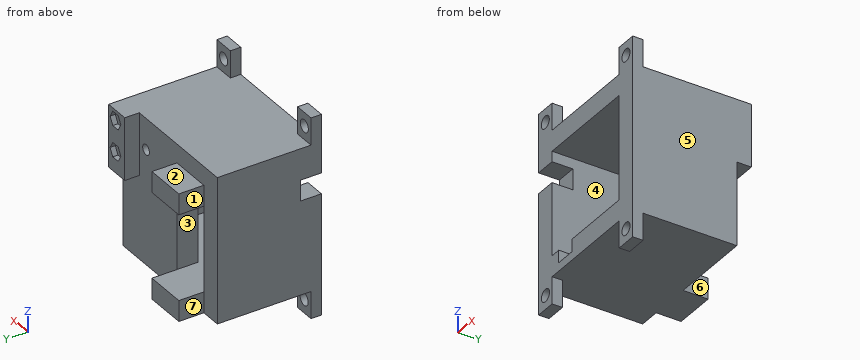
from build123d import *

# Parameters (mm, degrees)
SKETCH1_W               = 70
SKETCH1_H               = 70
BOSS_EXTRUDE1_DEPTH     = 50
CUT_EXTRUDE1_DEPTH      = 40
SKETCH3_W               = 20
SKETCH3_H               = 41
CUT_EXTRUDE2_DEPTH      = 40
SKETCH4_W               = 12
SKETCH4_H               = 30
BOSS_EXTRUDE2_DEPTH     = 7
CUT_EXTRUDE3_DEPTH      = 2.5
SKETCH7_R               = 2.5
CUT_EXTRUDE4_DEPTH      = 52.5
CUT_EXTRUDE5_DEPTH      = 97.81941954
CUT_EXTRUDE5_DEPTH_BACK = 52.5
SKETCH9_W               = 10
SKETCH9_H               = 10
SKETCH10_W              = 10
SKETCH10_H              = 6
CUT_EXTRUDE6_DEPTH      = 35
SKETCH11_W              = 20
SKETCH11_H              = 10
BOSS_EXTRUDE3_DEPTH     = 12
SKETCH13_W              = 10
SKETCH13_H              = 5
BOSS_EXTRUDE4_DEPTH     = 13
SKETCH14_W              = 10
SKETCH14_H              = 5
BOSS_EXTRUDE5_DEPTH     = 13
SKETCH15_R              = 3
CUT_EXTRUDE7_DEPTH      = 33


with BuildPart() as part:
    # Sketch1 → Boss-Extrude1 (new body)
    with BuildSketch(Plane(origin=(0, 0, 0), x_dir=(1, 0, 0), z_dir=(0, 1, 0))):
        Rectangle(SKETCH1_W, SKETCH1_H)
    extrude(amount=BOSS_EXTRUDE1_DEPTH)

    # Sketch2 → Cut-Extrude1 (cut)
    with BuildSketch(Plane.XZ):
        Polygon((0, 25), (-25, 25), (-25, -25), (25, -25), (25, 25), align=None)
    extrude(amount=-CUT_EXTRUDE1_DEPTH, mode=Mode.SUBTRACT)

    # Sketch3 → Cut-Extrude2 (cut)
    with BuildSketch(Plane(origin=(0, 50, 0), x_dir=(1, 0, 0), z_dir=(0, 1, 0))):
        with Locations((-15, 4.5)):
            Rectangle(SKETCH3_W, SKETCH3_H)
    extrude(amount=-CUT_EXTRUDE2_DEPTH, mode=Mode.SUBTRACT)

    # Sketch4 → Boss-Extrude2 (add)
    with BuildSketch(Plane(origin=(0, 50, 0), x_dir=(1, 0, 0), z_dir=(0, 1, 0))):
        with Locations((29, -20)):
            Rectangle(SKETCH4_W, SKETCH4_H)
    extrude(amount=BOSS_EXTRUDE2_DEPTH)

    # Sketch5 → Cut-Extrude3 (cut)
    with BuildSketch(Plane(origin=(0, 57, 0), x_dir=(1, 0, 0), z_dir=(0, 1, 0))):
        Polygon((33.881686691, -15), (31.881686691, -18.464101615), (27.881686691, -18.464101615), (25.881686691, -15), (27.881686691, -11.535898385), (31.881686691, -11.535898385), align=None)
        Polygon((27.881686691, -33.464101615), (25.881686691, -30), (27.881686691, -26.535898385), (31.881686691, -26.535898385), (33.881686691, -30), (31.881686691, -33.464101615), align=None)
    extrude(amount=-CUT_EXTRUDE3_DEPTH, mode=Mode.SUBTRACT)

    # Sketch7 → Cut-Extrude4 (cut)
    with BuildSketch(Plane(origin=(0, 50, 0), x_dir=(1, 0, 0), z_dir=(0, 1, 0))):
        with Locations(Location((18, -20, 0), (0, 0, 270))):
            Circle(SKETCH7_R)
    extrude(amount=-CUT_EXTRUDE4_DEPTH, mode=Mode.SUBTRACT)

    # Sketch9 → Cut-Extrude5 (cut, two sides: drawn at the far end of the back side and taken through both)
    with BuildSketch(Plane.ZY.offset(35).offset(-CUT_EXTRUDE5_DEPTH_BACK)):
        with Locations((15, 5)):
            Rectangle(SKETCH9_W, SKETCH9_H)
    extrude(amount=CUT_EXTRUDE5_DEPTH + CUT_EXTRUDE5_DEPTH_BACK, mode=Mode.SUBTRACT)

    # Sketch10 → Cut-Extrude6 (cut)
    with BuildSketch(Plane.XZ):
        with Locations((-15, -28)):
            Rectangle(SKETCH10_W, SKETCH10_H)
    extrude(amount=-CUT_EXTRUDE6_DEPTH, mode=Mode.SUBTRACT)

    # Sketch11 → Boss-Extrude3 (add)
    with BuildSketch(Plane(origin=(0, 50, 0), x_dir=(1, 0, 0), z_dir=(0, 1, 0))):
        with Locations((-15, 30)):
            Rectangle(SKETCH11_W, SKETCH11_H)
        with Locations((-15, -21)):
            Rectangle(SKETCH11_W, SKETCH11_H)
    extrude(amount=BOSS_EXTRUDE3_DEPTH)

    # Sketch13 → Boss-Extrude4 (add)
    with BuildSketch(Plane.XY.offset(35)):
        with Locations((-30, 2.5)):
            Rectangle(SKETCH13_W, SKETCH13_H)
        with Locations((30, 2.5)):
            Rectangle(SKETCH13_W, SKETCH13_H)
    extrude(amount=BOSS_EXTRUDE4_DEPTH)

    # Sketch14 → Boss-Extrude5 (add)
    with BuildSketch(Plane(origin=(0, 0, -35), x_dir=(-1, 0, 0), z_dir=(0, 0, -1))):
        with Locations((-30, 2.5)):
            Rectangle(SKETCH14_W, SKETCH14_H)
        with Locations((30, 2.5)):
            Rectangle(SKETCH14_W, SKETCH14_H)
    extrude(amount=BOSS_EXTRUDE5_DEPTH)

    # Sketch15 → Cut-Extrude7 (cut)
    with BuildSketch(Plane(origin=(0, 5, 0), x_dir=(1, 0, 0), z_dir=(0, 1, 0))):
        with Locations(Location((-29.888443239, 41.354976211, 0), (0, 0, 180))):
            Circle(SKETCH15_R)
        with Locations(Location((-30, -41.5, 0), (0, 0, 180))):
            Circle(SKETCH15_R)
        with Locations(Location((30, -41.5, 0), (0, 0, 180))):
            Circle(SKETCH15_R)
        with Locations(Location((30, 41.5, 0), (0, 0, 180))):
            Circle(SKETCH15_R)
    extrude(amount=-CUT_EXTRUDE7_DEPTH, mode=Mode.SUBTRACT)


solid = part.part
Read the model definition and answer for the solid it produces. Units are mm, in the model's axes. Face numbers are marked on the shaded views. A direction names the side the tool comes from. Give positions to 0.01 mm unless a question says otherwise; leave off trailing zeros. Loops run counter-clockwise (first coordinate to the right, second up) from the corner with the lowest first, then second, coordinate; pieces in that order, holes last. Notation, with made-up numbers: M 8.25,2.5 L 30.25,2.5 A15 ccw 30.25,31.5 Z; hole C -28,72 d10. An arc over 180 degrees is marked long. Write each question's results on one line, items separated by ' | '.
1. Given pin 1 (3 mm diameter, centred on x = -2, y = 16.5, fed in from -Z); pin 2 (8 mm diameter, centred on x = -12, z = 34, fed in from +Y); pin 3 (10 mm diameter, centred on x = 15.5, y = 52.5, fed in from +Z), each flat-ended and moving along its own axis, determine where each tip first touches the part or whether it passes through.
Values:
pin 1: stops at z = -35 | pin 2: stops at y = 50 | pin 3: stops at z = 35
2. Section C-C on x = -7.5 is taken. Give the vertices of the cut face in (y, z), plus the area to 3 significant figures.
Values:
outline: M 0,-35 L 62,-35 L 62,-25 L 0,-25 Z; M 0,25 L 40,25 L 40,16 L 62,16 L 62,26 L 50,26 L 50,35 L 0,35 Z | area: 1,330 mm^2
3. Section D-D on y = 13 is taken. Give the vertices of the cut face in (x, z).
Values:
outline: M -35,-35 L 35,-35 L 35,35 L -35,35 Z; hole M -25,-25 L -20,-25 L -20,-31 L -10,-31 L -10,-25 L 25,-25 L 25,25 L -25,25 Z
4. Straight lines are drawn through the part: line 1 (Z direction, x = 30, y = 1); line 2 (X direction, y = 39.5, z = 16); line 3 (X direction, y = 34, z = -30). For each, find the intervals that lie inside material, in ascending order. Write a range as [from, to].
Values:
line 1: z = [-48, -44.5], [-38.5, 38.5], [44.5, 48] | line 2: x = [-35, -25], [25, 35] | line 3: x = [-35, -20], [-10, 35]
5. A tool of negligible diameter and unlimited length cuts with its end or side. For the marked faces 4, 5, 6 and 7, from which of +Z, -Z, +X, -X, +Y, -Y can it reach the whole face along a straight path? Write none if from no direction.
Values:
face 4: -Y | face 5: +Z, -Z, +X, +Y, -Y | face 6: +Z, -Z, +X, +Y | face 7: +Z, -Z, -X, +Y
6. Section A-A on z = -15 is taken. Give the vertices of the cut face in (x, y).
Values:
outline: M -35,0 L -25,0 L -25,50 L -35,50 Z; M -5,40 L 25,40 L 25,0 L 35,0 L 35,50 L -5,50 Z
7. Section B-B on y = 53 is taken. Give the vertices of the cut face in (x, z), plus the area to 3 significant figures.
Values:
outline: M -25,-35 L -5,-35 L -5,-25 L -25,-25 Z; M -25,16 L -5,16 L -5,26 L -25,26 Z; M 23,5 L 35,5 L 35,35 L 23,35 Z | area: 760 mm^2
8. The mould has two halves that part along Z. Classify the marked faces 1, 2 and 3: pulls with the +Z half, pulls with the -Z half, needs draft (parallel to the pull), parting line crosses it, or undercut.
Values:
face 1: needs draft | face 2: pulls with the +Z half | face 3: undercut
